Answer from the drawing. Dimensions are ordinates in mm from the lowest x, y and z of the part. Give positions to 0.01 mm unless a question says otherwise; leave off trailing zeros. Write each loop counter-clockwise with the first axis right and the second up, starting at its lowest first coordinate (ties: lowest second). Pieces come first, ordered by that corner, then holes. Notation, with made-up numbers: (63.25, -12) -> (70.25, -12) arc R20 cw to (70.25, -6) -> close; hole circle Ø8 at (53.5, 39). An arc over 180 degrees is marked (long way). Use a Markdown table: item, result. Add a question column.
Q1. Section A-A, the plane y = 23 is taken. Give the vertices of the cut face in (x, z), plus the area to 3 significant figures.
Q2. Section D-D, the plane y = 34 is taken. Give the vertices of the cut face in (x, z).
Q3. This flat-tipped pin is pushed along its axis until it touches: pin 1 Ø7 at (x, y) = (74.5, 36.15) entering from +Z. Where does it stop, or does it pass through?
Q4. Consider line 1 (Y direction, x = 74.5, z = 1.9); line 2 (X direction, y = 19.5, z = 1.65); line 3 (X direction, y = 25.5, z = 0.9). Determine where each line is inside the solid, lowest interval first.
Q5. Section C-C, the plane z = 1.3 is taken. Give the vertices of the cut face in (x, y).
Q6. Section B-B, the plane x = 74.5 is taken. Give the vertices of the cut face in (y, z).
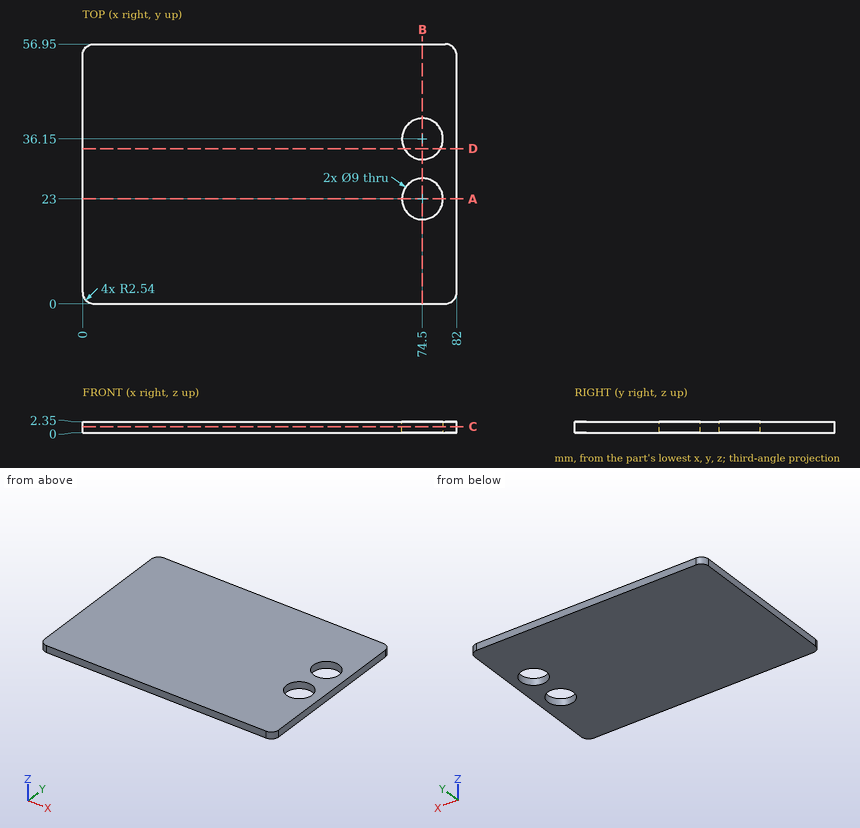
Result set:
| question | item | result |
|---|---|---|
| 1 | outline | (0, 0) -> (70, 0) -> (70, 2.35) -> (0, 2.35) -> close; (79, 0) -> (82, 0) -> (82, 2.35) -> (79, 2.35) -> close |
| 1 | area | 172 mm2 |
| 2 | outline | (0, 0) -> (70.55, 0) -> (70.55, 2.35) -> (0, 2.35) -> close; (78.45, 0) -> (82, 0) -> (82, 2.35) -> (78.45, 2.35) -> close |
| 3 | pin 1 | passes through |
| 4 | line 1 | y = 0 to 18.5, 27.5 to 31.65, 40.65 to 56.95 |
| 4 | line 2 | x = 0 to 71.67, 77.33 to 82 |
| 4 | line 3 | x = 0 to 70.76, 78.24 to 82 |
| 5 | outline | (0, 2.54) arc R2.54 ccw to (2.54, 0) -> (79.46, 0) arc R2.54 ccw to (82, 2.54) -> (82, 54.41) arc R2.54 ccw to (79.46, 56.95) -> (2.54, 56.95) arc R2.54 ccw to (0, 54.41) -> close; hole circle Ø9 at (74.5, 23); hole circle Ø9 at (74.5, 36.15) |
| 6 | outline | (0, 0) -> (18.5, 0) -> (18.5, 2.35) -> (0, 2.35) -> close; (27.5, 0) -> (31.65, 0) -> (31.65, 2.35) -> (27.5, 2.35) -> close; (40.65, 0) -> (56.95, 0) -> (56.95, 2.35) -> (40.65, 2.35) -> close |
